Source: CAD feature listing. Evaluate the final solid. Frame: model axes, mm. Give positions to 0.01 mm unless a question says otherwise; leave off trailing zeros. Loops run counter-clockwise (first coordinate to the right, second up) from the corner with the lowest first, then second, coordinate; pieces in that order, holes last. Notation, with made-up numbers: M 60.5,65 L 109.5,65 A19 cw 109.5,95 Z; hole C 0.5,68 d8. An arc over 180 degrees is marked long. Answer in a Markdown table with one row per item.
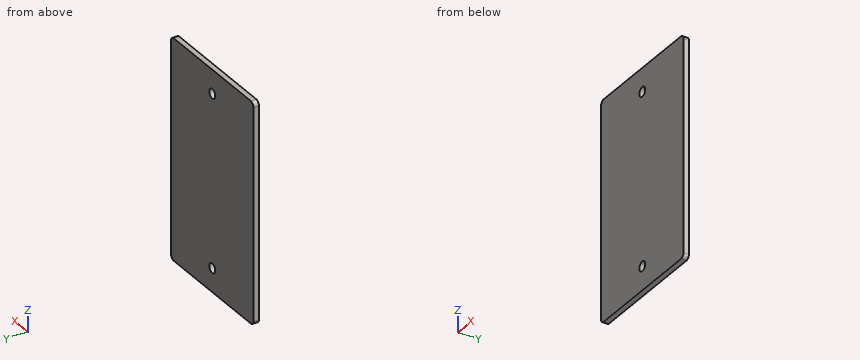
```python
from build123d import *

# Parameters (mm, degrees)
SKETCH1_W           = 76.2
SKETCH1_H           = 127
SKETCH1_R           = 2.75
BOSS_EXTRUDE1_DEPTH = 3.175
FILLET1_R           = 2.5


with BuildPart() as part:
    # Sketch1 → Boss-Extrude1 (new body)
    with BuildSketch(Plane(origin=(0, 0, 0), x_dir=(1, 0, 0), z_dir=(0, 1, 0))):
        Rectangle(SKETCH1_W, SKETCH1_H)
        with Locations((0, 49.785)):
            Circle(SKETCH1_R, mode=Mode.SUBTRACT)
        with Locations((0, -49.785)):
            Circle(SKETCH1_R, mode=Mode.SUBTRACT)
    extrude(amount=BOSS_EXTRUDE1_DEPTH)

    # Fillet1
    fillet1_edges = [part.edges().sort_by_distance(p)[0] for p in [
        (38.1, 1.5875, 63.5),
        (-38.1, 1.5875, 63.5),
        (-38.1, 1.5875, -63.5),
        (38.1, 1.5875, -63.5),
    ]]
    fillet(fillet1_edges, radius=FILLET1_R)


solid = part.part
```
1) Section A-A, the plane x = 0. Return loops of the section in (y, z) (3 decimals), then the cut area to 3 significant figures.
Reply:
| item | result |
|---|---|
| outline | M 0,-63.5 L 3.175,-63.5 L 3.175,-52.535 L 0,-52.535 Z; M 0,-47.035 L 3.175,-47.035 L 3.175,47.035 L 0,47.035 Z; M 0,52.535 L 3.175,52.535 L 3.175,63.5 L 0,63.5 Z |
| area | 368 mm² |
2) Pin query (flat end, axial travel): pin 1 Ø5 at (x, z) = (0, 49.785) entering from +Y. Return the tip coordinate at first contact, or that it passes through.
Reply:
| item | result |
|---|---|
| pin 1 | passes through |
3) Material intervals for L1, parallel to Z at x = 0, y = 1.4 (3 decimals); L2, parallel to X at y = 2, z = 50.5, sorted ascending.
Reply:
| item | result |
|---|---|
| L1 | z = -63.5 to -52.535, -47.035 to 47.035, 52.535 to 63.5 |
| L2 | x = -38.1 to -2.66, 2.66 to 38.1 |
